from build123d import *

# Parameters (mm, degrees)
BOSS_EXTRUDE1_DEPTH   = 10
BOSS_EXTRUDE1_2_DEPTH = 10
BOSS_EXTRUDE2_DEPTH   = 5
BOSS_EXTRUDE3_DEPTH   = 5


with BuildPart() as part:
    # Sketch1 → Boss-Extrude1 (new body)
    with BuildSketch(Plane.XY):
        with BuildLine():
            ThreePointArc((36.063682392, 40.248355648), (41.058703517, 28.189307903), (42.762412203, 15.248355648))
            Line((42.762412203, 15.248355648), (47.762412203, 15.248355648))
            ThreePointArc((47.762412203, 15.248355648), (45.888332649, 29.483403128), (40.393809411, 42.748355648))
            Line((40.393809411, 42.748355648), (36.063682392, 40.248355648))
        make_face()
    extrude(amount=BOSS_EXTRUDE1_DEPTH)



with BuildPart() as body_2:
    # Sketch1 → Boss-Extrude1 2 (new body)
    with BuildSketch(Plane.XY):
        with BuildLine():
            ThreePointArc((57.714317487, 52.748355648), (65.206849175, 34.65978403), (67.762412203, 15.248355648))
            Line((67.762412203, 15.248355648), (72.762412203, 15.248355648))
            ThreePointArc((72.762412203, 15.248355648), (70.036478306, 35.953879256), (62.044444506, 55.248355648))
            Line((62.044444506, 55.248355648), (57.714317487, 52.748355648))
        make_face()
    extrude(amount=BOSS_EXTRUDE1_2_DEPTH)


with BuildPart() as part_1:
    add(part.part)

    add(body_2.part)  # Boss-Extrude2 merges body 2
    # Sketch2 → Boss-Extrude2 (add)
    with BuildSketch(Plane.XY.offset(10)):
        with BuildLine():
            Line((36.063682392, 40.248355648), (62.044444506, 55.248355648))
            ThreePointArc((62.044444506, 55.248355648), (70.036478306, 35.953879256), (72.762412203, 15.248355648))
            Line((72.762412203, 15.248355648), (42.762412203, 15.248355648))
            ThreePointArc((42.762412203, 15.248355648), (41.058703517, 28.189307903), (36.063682392, 40.248355648))
        make_face()
    extrude(amount=BOSS_EXTRUDE2_DEPTH)

    # Sketch3 → Boss-Extrude3 (add)
    with BuildSketch(Plane(origin=(0, 0, 0), x_dir=(-1, 0, 0), z_dir=(0, 0, -1))):
        with BuildLine():
            Line((-36.063682392, 40.248355648), (-62.044444506, 55.248355648))
            ThreePointArc((-62.044444506, 55.248355648), (-70.036478306, 35.953879256), (-72.762412203, 15.248355648))
            Line((-72.762412203, 15.248355648), (-42.762412203, 15.248355648))
            ThreePointArc((-42.762412203, 15.248355648), (-41.058703517, 28.189307903), (-36.063682392, 40.248355648))
        make_face()
    extrude(amount=BOSS_EXTRUDE3_DEPTH)


solid = part_1.part
Can you work these out from the model? Positions are in its coordinate system, mm. A direction names the side the tool comes from. Coordinates: 2 decimals unless noted, no trailing zeros. Write each loop counter-clockwise with the first axis right and the second up, starting at its lowest first coordinate (ties: lowest second). Pieces come first, ordered by that corner, then holes. Notation, with made-up numbers: M -19,66 L 1,66 A22 cw 1,90 Z; hole C 85,-12.5 d5. An arc over 180 degrees is marked long. Use one line per item in the form item = value.
Q1. For P1, Ø1, axis at y = 41, z = 5, coming from the +X side; P2, Ø6, axis at x = 44, z = 8, coming from the +Y side; P3, Ø10, axis at y = 32.5, z = -0.5, coming from the +X side, each with a flat end and sliding along its axis, tell me the tip position at first contact or that it passes through.
Model answer:
P1 = 68.67
P2 = 46.12
P3 = 71.82
Q2. If we section it at B-B (x = 56.5): Write out the boundary of the cut face in (y, z), then the cut area to 3 significant figures.
Model answer:
outline = M 15.25,-5 L 52.05,-5 L 52.05,0 L 15.25,0 Z; M 15.25,10 L 52.05,10 L 52.05,15 L 15.25,15 Z
area = 368 mm^2
Q3. If we section it at A-A (z = 7.5): Write out the boundary of the cut face in (x, y), then the cut area to 3 significant figures.
Model answer:
outline = M 36.06,40.25 A50 cw 42.76,15.25 L 47.76,15.25 A55 ccw 40.39,42.75 Z; M 57.71,52.75 A75 cw 67.76,15.25 L 72.76,15.25 A80 ccw 62.04,55.25 Z
area = 340 mm^2
Q4. For faces 1 (the cylindrical face through (65.135, 34.925, 4.93)), 2 (the flat face through (48.87, 47.64, 11.81)), 3 (the cylindrical face through (45.94, 29.29, 4.93)), which set-ups out of +Z, -Z, +X, -X, +Y, -Y let a thin tool reach every point of the face, with its end or its side?
Model answer:
face_1 = -Y
face_2 = +Z, -Z, -X, +Y
face_3 = +Y
Q5. If we section it at D-D (z = -2.25): Write out the boundary of the cut face in (x, y), then the cut area to 3 significant figures.
Model answer:
outline = M 36.06,40.25 A50 cw 42.76,15.25 L 72.76,15.25 A80 ccw 62.04,55.25 Z
area = 1,020 mm^2
Q6. I need wall thicknesses on line 1 along Z through (x, y) = (57.5, 49); line 2 along X through (y, z) = (24.5, 8); line 3 along X through (y, z) = (27.5, 0.5). Which ranges of each line are inside material? Lowest first, please. Write a range as from..to.
Model answer:
line_1 = -5..0, 10..15
line_2 = 41.9..46.98, 67.19..72.23
line_3 = 41.24..46.38, 66.75..71.82
Q7. We'd pull the mould along Z, two halves only. Please class faces 4 (the cylindrical face through (41.106, 28.012, 5.14)), 5 (the flat face through (54, 30, 10)), 6 (the flat face through (55, 31, -5)): +Z half, -Z half, draft (parallel to the pull), parting line (faces both ways), or undercut.
Model answer:
face_4 = draft
face_5 = undercut
face_6 = -Z half
Q8. If we section it at C-C (y = 31): Write out the boundary of the cut face in (x, z), then the cut area to 3 significant figures.
Model answer:
outline = M 40.22,-5 L 71.2,-5 L 71.2,15 L 40.22,15 Z; hole M 45.46,0 L 66.09,0 L 66.09,10 L 45.46,10 Z
area = 413 mm^2
